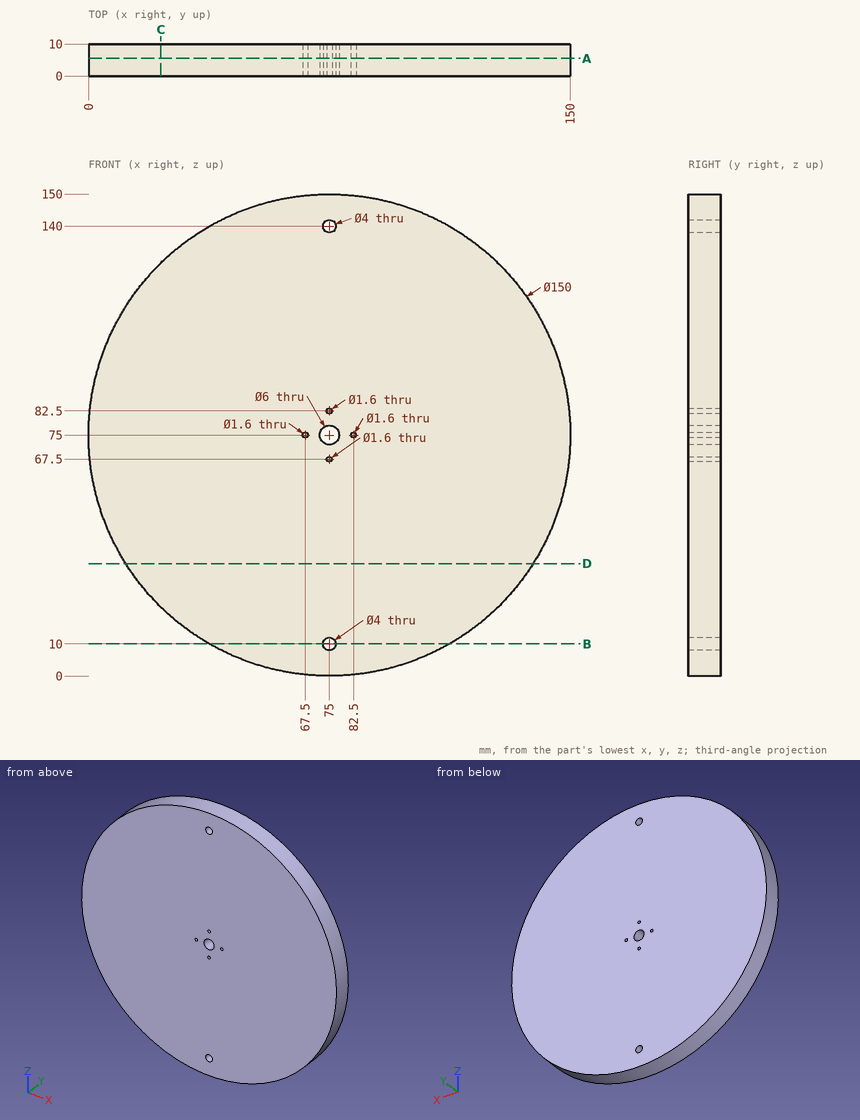
For this review, use the dimensioned drawing (mm, ordinates from the lowest corner) and the shaded views. Round coordinates to 2 decimals unless told otherwise and drop trailing zeros. Order: outer loops, then holes, each group sorted by start corner. A loop starts at its lowest first (then second) coordinate and runs counter-clockwise, first axis right, second up. Notation, with made-up numbers: (1, 17.25) - (32, 17.25) arc R27 ccw to (32, 45.25) - close; hole circle Ø2 at (-0.75, -27). An arc over 180 degrees is marked (long way). Use one line per item in the form item = value.
Q1. Clearance check with flat-ended pins moving along their axes: P1, Ø4, axis at x = 81, y = 4.5, coming from the -Z side; P2, Ø1.5, axis at x = 26.5, y = 4.5, coming from the -Z side; P3, Ø5, axis at x = 65.5, y = 5, coming from the -Z side; P4, Ø1.4, axis at x = 82.5, z = 75, coming from the -Y side. State where each tip first meets the part, or that it passes through.
Response values:
P1 = 0.11
P2 = 17.16
P3 = 0.33
P4 = through
Q2. To check wall thickness, follow line 1 (X direction, y = 2, z = 75); line 2 (X direction, y = 5.75, z = 140); line 3 (Z direction, x = 67.5, y = 6.75). State the ranges of each line that lie inside material, in increasing order.
Response values:
line_1 = 0 to 66.7, 68.3 to 72, 78 to 81.7, 83.3 to 150
line_2 = 37.58 to 73, 77 to 112.42
line_3 = 0.38 to 74.2, 75.8 to 149.62
Q3. Add section B-B on z = 10. Give the boundary of the cut face in (x, y).
Response values:
outline = (37.58, 0) - (73, 0) - (73, 10) - (37.58, 10) - close; (77, 0) - (112.42, 0) - (112.42, 10) - (77, 10) - close
Q4. Add section D-D on z = 35. Give the boundary of the cut face in (x, y).
Response values:
outline = (11.56, 0) - (138.44, 0) - (138.44, 10) - (11.56, 10) - close
Q5. Add section A-A on y = 5.5. Give the boundary of the cut face in (x, z), then the cut area to 3 significant figures.
Response values:
outline = circle Ø150 at (75, 75); hole circle Ø1.6 at (67.5, 75); hole circle Ø6 at (75, 75); hole circle Ø4 at (75, 10); hole circle Ø4 at (75, 140); hole circle Ø1.6 at (75, 67.5); hole circle Ø1.6 at (75, 82.5); hole circle Ø1.6 at (82.5, 75)
area = 17,600 mm^2
Q6. Add section C-C on x = 22.5. Give the boundary of the cut face in (y, z).
Response values:
outline = (0, 21.44) - (10, 21.44) - (10, 128.56) - (0, 128.56) - close
